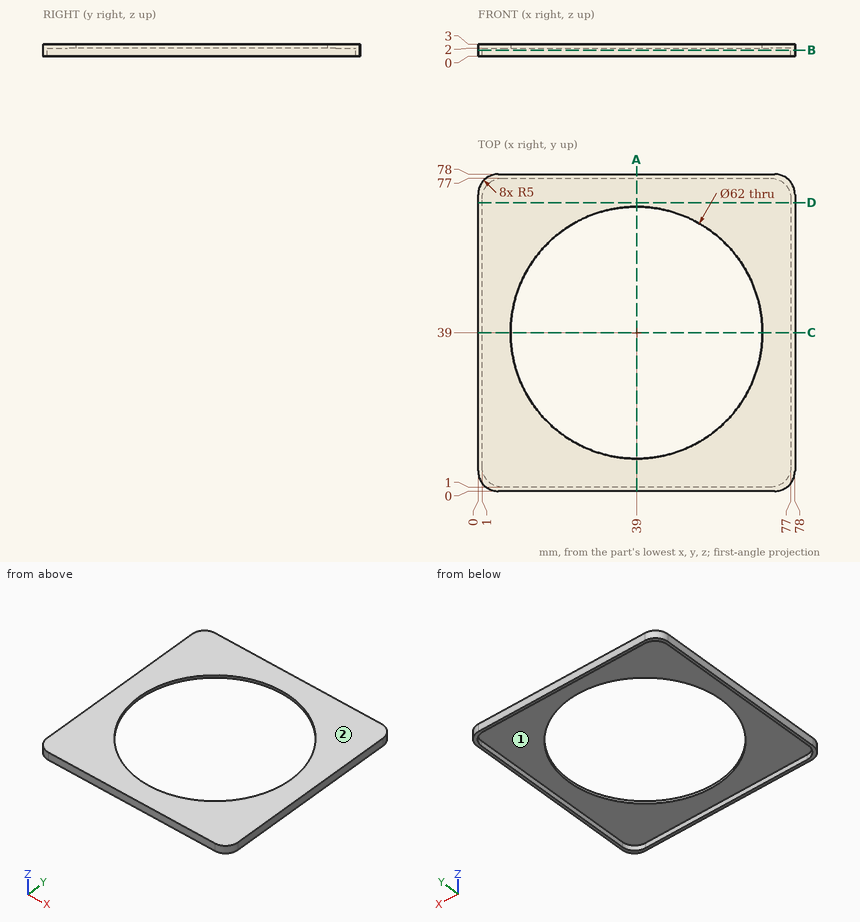
Study the drawing (mm; zero at the part's minimum x, y, z) and answer. Give positions to 0.01 mm unless a question says otherwise; leave off trailing zeros. Order: outer loops, then holes, each group sorted by start corner. A loop starts at its lowest first (then second) coordinate and runs counter-clockwise, first axis right, second up. Notation, with made-up numbers: (23, -6.5) -> (65, -6.5) arc R10 cw to (65, 0.5) -> close; hole circle Ø8 at (80, 1.5). An arc over 180 degrees is marked (long way). Put each result on its own line as item: value.
Item 1: A cutting plane is placed at B-B on z = 1.5. Give the vertices of the cut face in (x, y).
Established:
outline: (0, 5) arc R5 ccw to (5, 0) -> (73, 0) arc R5 ccw to (78, 5) -> (78, 73) arc R5 ccw to (73, 78) -> (5, 78) arc R5 ccw to (0, 73) -> close; hole (1, 6) arc R5 ccw to (6, 1) -> (72, 1) arc R5 ccw to (77, 6) -> (77, 72) arc R5 ccw to (72, 77) -> (6, 77) arc R5 ccw to (1, 72) -> close
Item 2: A cutting plane is placed at D-D on y = 71. Give the vertices of the cut face in (x, z).
Established:
outline: (0, 0) -> (1, 0) -> (1, 2) -> (77, 2) -> (77, 0) -> (78, 0) -> (78, 3) -> (0, 3) -> close
Item 3: Given P1, Ø23, axis at x = 55.5, y = 20, coming from the -Z side, flat-ended and moving along its own axis, determine where the tip first touches the part or whether it passes through.
Established:
P1: stops at z = 2
Item 4: Straight lines are drawn through the part: line 1 (X direction, y = 16, z = 1.7); line 2 (Y direction, x = 39, z = 2.65). For each, find the intervals that lie inside material, in ascending order.
Established:
line 1: x = 0 to 1, 77 to 78
line 2: y = 0 to 8, 70 to 78
Item 5: A cutting plane is placed at A-A on x = 39. Give the vertices of the cut face in (y, z).
Established:
outline: (0, 0) -> (1, 0) -> (1, 2) -> (8, 2) -> (8, 3) -> (0, 3) -> close; (70, 2) -> (77, 2) -> (77, 0) -> (78, 0) -> (78, 3) -> (70, 3) -> close
Item 6: For a pull along Y with two mould halves and no side action, classify the marked faces 1 and 2 as released by +Y, released by -Y, zero draft, split by the parting line, or undercut.
Established:
face 1: undercut
face 2: zero draft
